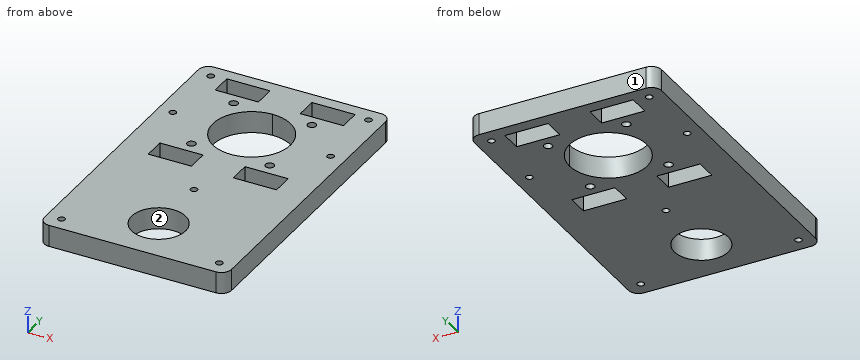
from build123d import *

# Parameters (mm, degrees)
F0_W     = 55
F0_H     = 90
F0_W_2   = 12.7
F0_H_2   = 6.35
F1_DEPTH = 6.35
F2_D     = 2.5
F3_R     = 3
F4_D     = 15.83
F5_D     = 2


with BuildPart() as f1:
    # F0 (on Top) → F1 (new body)
    with BuildSketch(Plane.XY):
        with Locations((0, -20)):
            Rectangle(F0_W, F0_H)
        with Locations((-12.5, -18.25)):
            Rectangle(F0_W_2, F0_H_2, mode=Mode.SUBTRACT)
        with Locations((-12.5, 18.25)):
            Rectangle(F0_W_2, F0_H_2, mode=Mode.SUBTRACT)
        with Locations((12.5, -18.25)):
            Rectangle(F0_W_2, F0_H_2, mode=Mode.SUBTRACT)
        with BuildLine():
            ThreePointArc((0, 11.4), (8.0610173055, 8.0610173055), (11.4, 0))
            ThreePointArc((11.4, 0), (-8.0610173055, -8.0610173055), (0, 11.4))
        make_face(mode=Mode.SUBTRACT)
        with Locations((12.5, 18.25)):
            Rectangle(F0_W_2, F0_H_2, mode=Mode.SUBTRACT)
    extrude(amount=F1_DEPTH)

    # F2 (through all)
    with Locations(Plane(origin=(0, 0, 0), x_dir=(1, 0, 0), z_dir=(0, 0, -1))):
        with Locations((-11.5, -11.5), (11.5, -11.5), (11.5, 11.5), (-11.5, 11.5)):
            Hole(F2_D / 2)

    # F3
    f3_edges = [f1.edges().sort_by_distance(p)[0] for p in [
        (-27.5, -65, 3.175),
        (27.5, -65, 3.175),
        (27.5, 25, 3.175),
        (-27.5, 25, 3.175),
    ]]
    fillet(f3_edges, radius=F3_R)

    # F4 (through all)
    with Locations(Plane(origin=(0, 0, 0), x_dir=(1, 0, 0), z_dir=(0, 0, -1))):
        with Locations((0, 50.735)):
            Hole(F4_D / 2)

    # F5 (through all)
    with Locations(Plane(origin=(0, 0, 0), x_dir=(1, 0, 0), z_dir=(0, 0, -1))):
        with Locations((-23.175, -20.675), (23.175, -20.675), (23.175, 0), (-23.175, 0), (-23.175, 60.675), (23.175, 60.675), (0, 31.431786716)):
            Hole(F5_D / 2)


solid = f1.part
For this review, take the finished solid that the model builds, in its own axes (mm). Face numbers are marked on the shaded views. Round coordinates to 2 decimals unless told otherwise and drop trailing zeros. Write each loop counter-clockwise with the first axis right and the second up, starting at its lowest first coordinate (ties: lowest second). Pieces come first, ordered by that corner, then holes. Notation, with made-up numbers: M 56,-36 L 94,-36 A27 cw 94,-15 Z; hole C 83,-3 d3. An arc over 180 degrees is marked long. Write item = value, one per line. Start each with the question number.
(1) We need section A-A (y = -19). Give the boundary of the cut face in (x, z).
(2) We need section C-C (z = 5.25). Give the number of separate pieces and of enclosed holes in the cut face, then the cut area to 3 significant figures.
(3) We need section B-B (x = -17.5). Give the boundary of the cut face in (y, z) (3 decimals).
(4) For line 1 along Y through (x, z) = (-14.5, 3.25) (3 decimals); line 2 along X through (y, z) = (-11.5, 4); line 3 along Y through (x, z) = (-11.5, 2.5) (3 decimals), list the stretches that pass through material, from the lowest coordinate up.
(5) Clearance check with a flat-ended pin moving along its axis: pin 1 Ø1.8 at (x, y) = (-23.175, 20.675) entering from +Z. State where the tip first meets the part, or that it passes through.
(6) The part is to be moulded in two halves that separate along X. For the marked faces 1 and 2, say which applies: +X half, -X half, draft (parallel to the pull), parting line (faces both ways), or undercut.
Results found:
q1.outline = M -27.5,0 L -18.85,0 L -18.85,6.35 L -27.5,6.35 Z; M -6.15,0 L 6.15,0 L 6.15,6.35 L -6.15,6.35 Z; M 18.85,0 L 27.5,0 L 27.5,6.35 L 18.85,6.35 Z
q2.separate_pieces = 1
q2.enclosed_holes = 17
q2.area = 3,970 mm²
q3.outline = M -65,0 L -21.425,0 L -21.425,6.35 L -65,6.35 Z; M -15.075,0 L 15.075,0 L 15.075,6.35 L -15.075,6.35 Z; M 21.425,0 L 25,0 L 25,6.35 L 21.425,6.35 Z
q4.line_1 = -65 to -21.425, -15.075 to 15.075, 21.425 to 25
q4.line_2 = -27.5 to -12.75, -10.25 to 10.25, 12.75 to 27.5
q4.line_3 = -65 to -21.425, -15.075 to -12.75, -10.25 to 10.25, 12.75 to 15.075, 21.425 to 25
q5.pin_1 = through
q6.face_1 = draft
q6.face_2 = undercut
